For this review, take the finished solid that the model builds, in its own axes (mm). Face numbers are marked on the shaded views. A direction names the side the tool comes from. Give positions to 0.01 mm unless a question says otherwise; leave off trailing zeros. Order: outer loops, then holes, each group sorted by start corner. A loop starts at its lowest first (then second) coordinate and runs counter-clockwise, first axis right, second up. Notation, with made-up numbers: (19, 25.25) - (37, 25.25) arc R15 cw to (37, 46.25) - close; hole circle Ø3 at (-9.75, 88.5). An arc over 180 degrees is marked (long way). Answer as a JSON object with one key per item and string values. Group by question number.
from build123d import *
from OCP.BRepFilletAPI import BRepFilletAPI_MakeChamfer

# Parameters (mm, degrees)
EXTRUDE_1_DEPTH     = 10
SKETCH_2_R          = 1.5
SKETCH_2_R_2        = 1.3
CUT_EXTRUDE_1_DEPTH = 46.08880127
CHAMFER_1_SIZE      = 3
CHAMFER_1_SIZE2     = 3.782343513
CHAMFER_1_SIZE2_2   = 2.562232702
CHAMFER_2_SIZE      = 2


with BuildPart() as part:
    # 草图1 → 凸台-拉伸1 (new body)
    with BuildSketch(Plane(origin=(0, 0, 0), x_dir=(1, 0, 0), z_dir=(0, 1, 0))):
        Polygon((13, -14.15), (5, -14.15), (5, -11), (-3.5, -11), (-3.5, 11), (5, 11), (5, 14.15), (13, 14.15), (13, 17.15), (5, 17.15), (5, 21), (-5, 21), (-5, 13), (-13, 13), (-13, 10), (-5, 10), (-5, -10), (-13, -10), (-13, -13), (-5, -13), (-5, -21), (5, -21), (5, -17.15), (13, -17.15), align=None)
    extrude(amount=EXTRUDE_1_DEPTH)

    # 草图2 → 切除-拉伸1 (cut, through all)
    with BuildSketch(Plane.XY.offset(21)):
        with Locations((10, 5)):
            Circle(SKETCH_2_R)
        with Locations((-8, 2.5)):
            Circle(SKETCH_2_R)
        with Locations((1.5, 3)):
            Circle(SKETCH_2_R_2)
        Polygon((-13, 5), (13, 10), (-13, 10), align=None)
    extrude(amount=-CUT_EXTRUDE_1_DEPTH, mode=Mode.SUBTRACT)

    # 倒角1: one chamfer whose edges measure the first distance from different faces: ONE call of the kernel's chamfer builder (chamfer() names one face for all edges)
    chamfer_1_edges_1 = [part.edges().sort_by_distance(p)[0] for p in [
        (-13, 5, -11.5),
    ]]
    chamfer_1_side_1 = [part.faces().sort_by_distance(p)[0] for p in [
        (-13, 2.5, -11.5),
    ]]
    chamfer_1_edges_2 = [part.edges().sort_by_distance(p)[0] for p in [
        (-13, 5, 11.5),
    ]]
    chamfer_1_side_2 = [part.faces().sort_by_distance(p)[0] for p in [
        (-13, 2.5, 11.5),
    ]]
    chamfer_1_edges_3 = [part.edges().sort_by_distance(p)[0] for p in [
        (13, 10, 15.65),
    ]]
    chamfer_1_side_3 = [part.faces().sort_by_distance(p)[0] for p in [
        (13, 5, 15.65),
    ]]
    chamfer_1_edges_4 = [part.edges().sort_by_distance(p)[0] for p in [
        (13, 10, -15.65),
    ]]
    chamfer_1_side_4 = [part.faces().sort_by_distance(p)[0] for p in [
        (-9, 5.769230769, 12.503512337),
    ]]
    chamfer_1 = BRepFilletAPI_MakeChamfer(part.part.solid().wrapped)
    for e in chamfer_1_edges_1:
        chamfer_1.Add(CHAMFER_1_SIZE, CHAMFER_1_SIZE2, e.wrapped, chamfer_1_side_1[0].wrapped)  # the first distance lies on this face
    for e in chamfer_1_edges_2:
        chamfer_1.Add(CHAMFER_1_SIZE, CHAMFER_1_SIZE2, e.wrapped, chamfer_1_side_2[0].wrapped)  # the first distance lies on this face
    for e in chamfer_1_edges_3:
        chamfer_1.Add(CHAMFER_1_SIZE, CHAMFER_1_SIZE2_2, e.wrapped, chamfer_1_side_3[0].wrapped)  # the first distance lies on this face
    for e in chamfer_1_edges_4:
        chamfer_1.Add(CHAMFER_1_SIZE, CHAMFER_1_SIZE2_2, e.wrapped, chamfer_1_side_4[0].wrapped)  # the first distance lies on this face
    add(Compound.cast(chamfer_1.Shape()), mode=Mode.REPLACE)

    # 倒角2
    chamfer_2_edges = [part.edges().sort_by_distance(p)[0] for p in [
        (0, 7.5, -21),
        (0.75, 7.644230769, 11),
        (0.75, 7.644230769, -11),
        (0, 7.5, 21),
    ]]
    chamfer(chamfer_2_edges, length=CHAMFER_2_SIZE)


solid = part.part
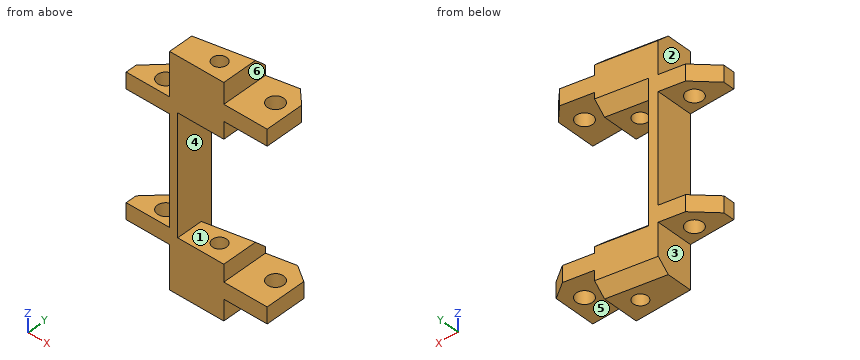
1) For line 1 (Z direction, x = 10.25, y = 1.5); line 2 (Z direction, x = -7, y = 4.25); line 3 (X direction, y = 1.25, z = 19), list the stretches that pass through material, from the lowest coordinate up.
2) Consider section C-C (x = 1.5). Give the boundary of the cut face in (y, z), plus the area to 3 significant figures.
3) Consider section A-A (z = 16). Give the boundary of the cut face in (x, y).
4) Mouldability with a two-part tool opening along Z and no side actions: class the marked faces 4, 5 and 6 as released by +Z, released by -Z, zero draft, split by the parting line, or undercut.
5) For the marked faces 1, 2 and 3, list the 3-axis set-ups (+Z, -Z, +X, -X, +Y, -Y) from which the entire face can be reached by the end or side of a thin tool; tool diameter is ignored.
6) Consider section D-D (y = 8). Give the boundary of the cut face in (x, z), plus the area to 3 significant figures.
7) For pin 1 (5 mm diameter, centred on x = -8, y = 2.5, fed in from -Z); pin 2 (2.5 mm diameter, centred on x = 7.5, y = 5, fed in from -Z); pin 3 (5.5 mm diameter, centred on y = 4.5, z = -3, fed in from +X); pin 4 (2.5 mm diameter, centred on x = 10, y = 5, fed in from -Z), all flat-tipped, find the tip position at first contact; note any pin that passes through.
8) Consider section B-B (x = -2). Give the boundary of the cut face in (y, z), plus the area to 3 significant figures.
Result set:
{
 "1": {"line 1": "z = -17.15 to -14.15, 14.15 to 17.15", "line 2": "z = -13 to -10, 10 to 13", "line 3": "x = -5 to 5"},
 "2": {"outline": "(0, -21) - (1.7, -21) - (1.7, -11) - (0, -11) - close; (0, 11) - (1.7, 11) - (1.7, 21) - (0, 21) - close; (4.3, -21) - (5.75, -21) - (7.79, -19) - (7.79, -13) - (5.75, -11) - (4.3, -11) - close; (4.3, 11) - (5.75, 11) - (7.79, 13) - (7.79, 19) - (5.75, 21) - (4.3, 21) - close", "area": "95.6 mm2"},
 "3": {"outline": "(-5, 0) - (13, 0) - (13, 7) - (10.48, 9.52) - (-5, 6.54) - close; hole circle Ø2.6 at (1.5, 3); hole circle Ø3 at (10, 5)"},
 "4": {"face 4": "undercut", "face 5": "released by -Z", "face 6": "zero draft"},
 "5": {"face 1": "+X, +Y, -Y", "face 2": "+Z, -X, +Y, -Y", "face 3": "-Z, -X, +Y, -Y"},
 "6": {"outline": "(2.6, -19) - (5, -19.45) - (5, -17.15) - (12.17, -17.15) - (12.17, -14.15) - (5, -14.15) - (5, -12.55) - (2.6, -13) - close; (2.6, 13) - (5, 12.55) - (5, 14.15) - (12, 14.15) - (12, 17.15) - (5, 17.15) - (5, 19.45) - (2.6, 19) - close", "area": "73.5 mm2"},
 "7": {"pin 1": "stops at z = -13", "pin 2": "stops at z = -17.15", "pin 3": "stops at x = -3.5", "pin 4": "passes through"},
 "8": {"outline": "(0, -21) - (5.08, -21) - (7.12, -19) - (7.12, -13) - (5.08, -11) - (0, -11) - close; (0, 11) - (5.08, 11) - (7.12, 13) - (7.12, 19) - (5.08, 21) - (0, 21) - close", "area": "134 mm2"}
}
